Check sheet for the modelled part. Datum: model origin and axes. Units: mm. Face numbers are marked on the shaded views. Round coordinates to 2 decimals unless told otherwise and drop trailing zeros. Loops run counter-clockwise (first coordinate to the right, second up) from the corner with the lowest first, then second, coordinate; pieces in that order, holes last. Notation, with made-up numbers: (74.5, -8.5) -> (131.5, -8.5) arc R27 cw to (131.5, 20.5) -> close; hole circle Ø5 at (-20.5, 52). An arc over 180 degrees is marked (long way). One line per item, written item: value. Start each with the question number.
1. Material ranges on L1, parallel to X at y = 9, z = -64; L2, parallel to X at y = -8.5, z = -61.5; L3, parallel to Y at x = -8, z = -107.95, recorded low to high.
2. Cross-section at A-A on y = 54. Record the cut outline in (x, z), then the cut area to 3 significant figures.
3. Cross-section at B-B on y = 9. Record the cut outline in (x, z).
4. Release check for a two-part mould opening along X. For the marked faces 1, 2 and 3 record: +X half, -X half, draft (parallel to the pull), parting line (faces both ways), or undercut.
5. Go/stop test with flat-tipped pins: pin 1 (3 mm diameter, centred on y = 31, z = -119, fed in from +X); pin 2 (10 mm diameter, centred on x = 241.3, y = 0, fed in from -Z); pin 3 (8 mm diameter, centred on y = 50.5, z = -40, fed in from +X). Record where each tip stops, or that it passes through.
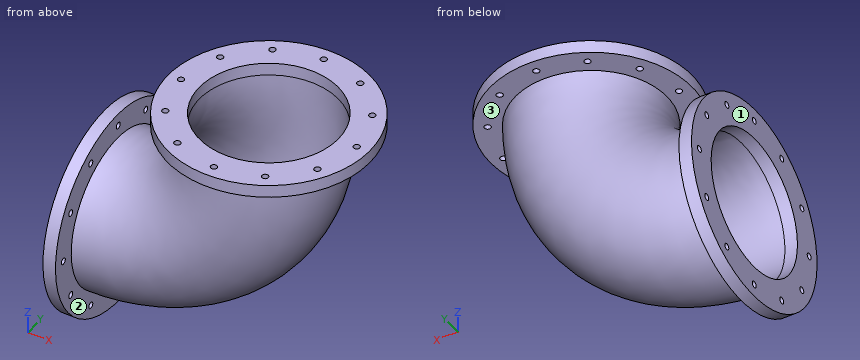
from build123d import *

# Parameters (mm, degrees)
SKETCH2_R           = 76.2
SKETCH2_R_2         = 69.85
SKETCH3_R           = 101.6
SKETCH3_R_2         = 69.85
SKETCH3_R_3         = 3.175
BOSS_EXTRUDE1_DEPTH = 12.7
SKETCH5_R           = 101.6
SKETCH5_R_2         = 69.85
SKETCH5_R_3         = 3.175
BOSS_EXTRUDE2_DEPTH = 12.7


with BuildPart() as part:
    # Sweep1: sweep along a path in Sketch1
    with BuildLine(Plane(origin=(0, 0, 0), x_dir=(1, 0, 0), z_dir=(0, 1, 0))) as sweep1_path:
        ThreePointArc((0, 152.4), (107.763073453, 107.763073453), (152.4, 0))
    # Sketch2 → Sweep1 (sweep)
    with BuildSketch(Plane(origin=(0, 0, 0), x_dir=(0, 0, -1), z_dir=(1, 0, 0))):
        with Locations((152.4, 0)):
            Circle(SKETCH2_R)
        with Locations((152.4, 0)):
            Circle(SKETCH2_R_2, mode=Mode.SUBTRACT)
    sweep(path=sweep1_path.line)

    # Sketch3 → Boss-Extrude1 (add)
    with BuildSketch(Plane.ZY):
        with Locations((-152.4, 0)):
            Circle(SKETCH3_R)
        with Locations((-152.4, 0)):
            Circle(SKETCH3_R_2, mode=Mode.SUBTRACT)
        with Locations((-241.3, 0)):
            Circle(SKETCH3_R_3, mode=Mode.SUBTRACT)
        with Locations((-229.389658396, -44.45)):
            Circle(SKETCH3_R_3, mode=Mode.SUBTRACT)
        with Locations((-196.85, -76.989658396)):
            Circle(SKETCH3_R_3, mode=Mode.SUBTRACT)
        with Locations((-152.4, -88.9)):
            Circle(SKETCH3_R_3, mode=Mode.SUBTRACT)
        with Locations((-107.95, -76.989658396)):
            Circle(SKETCH3_R_3, mode=Mode.SUBTRACT)
        with Locations((-75.410341604, -44.45)):
            Circle(SKETCH3_R_3, mode=Mode.SUBTRACT)
        with Locations((-63.5, 0)):
            Circle(SKETCH3_R_3, mode=Mode.SUBTRACT)
        with Locations((-75.410341604, 44.45)):
            Circle(SKETCH3_R_3, mode=Mode.SUBTRACT)
        with Locations((-107.95, 76.989658396)):
            Circle(SKETCH3_R_3, mode=Mode.SUBTRACT)
        with Locations((-152.4, 88.9)):
            Circle(SKETCH3_R_3, mode=Mode.SUBTRACT)
        with Locations((-196.85, 76.989658396)):
            Circle(SKETCH3_R_3, mode=Mode.SUBTRACT)
        with Locations((-229.389658396, 44.45)):
            Circle(SKETCH3_R_3, mode=Mode.SUBTRACT)
    extrude(amount=BOSS_EXTRUDE1_DEPTH)

    # Sketch5 → Boss-Extrude2 (add)
    with BuildSketch(Plane.XY):
        with Locations((152.4, 0)):
            Circle(SKETCH5_R)
        with Locations((152.4, 0)):
            Circle(SKETCH5_R_2, mode=Mode.SUBTRACT)
        with Locations((152.4, 88.9)):
            Circle(SKETCH5_R_3, mode=Mode.SUBTRACT)
        with Locations((196.85, 76.989658396)):
            Circle(SKETCH5_R_3, mode=Mode.SUBTRACT)
        with Locations((229.389658396, 44.45)):
            Circle(SKETCH5_R_3, mode=Mode.SUBTRACT)
        with Locations((241.3, 0)):
            Circle(SKETCH5_R_3, mode=Mode.SUBTRACT)
        with Locations((229.389658396, -44.45)):
            Circle(SKETCH5_R_3, mode=Mode.SUBTRACT)
        with Locations((196.85, -76.989658396)):
            Circle(SKETCH5_R_3, mode=Mode.SUBTRACT)
        with Locations((152.4, -88.9)):
            Circle(SKETCH5_R_3, mode=Mode.SUBTRACT)
        with Locations((107.95, -76.989658396)):
            Circle(SKETCH5_R_3, mode=Mode.SUBTRACT)
        with Locations((75.410341604, -44.45)):
            Circle(SKETCH5_R_3, mode=Mode.SUBTRACT)
        with Locations((63.5, 0)):
            Circle(SKETCH5_R_3, mode=Mode.SUBTRACT)
        with Locations((75.410341604, 44.45)):
            Circle(SKETCH5_R_3, mode=Mode.SUBTRACT)
        with Locations((107.95, 76.989658396)):
            Circle(SKETCH5_R_3, mode=Mode.SUBTRACT)
    extrude(amount=BOSS_EXTRUDE2_DEPTH)


solid = part.part
Taken from the geometry:
1. L1: x = -12.7 to 0, 42.33 to 53.06, 212.23 to 218.9
1. L2: x = -12.7 to 0, 45.79 to 55.84, 213.03 to 219.68
1. L3: y = -91.36 to -80.16, -73.81 to -53.88, 53.88 to 73.81, 80.16 to 91.36
2. outline: (-12.7, -238.46) -> (0, -238.46) -> (0, -206.16) arc R206.16 ccw to (206.16, 0) -> (238.46, 0) -> (238.46, 12.7) -> (196.71, 12.7) -> (196.71, 0) arc R196.71 cw to (0, -196.71) -> (-12.7, -196.71) -> close; (-12.7, -108.09) -> (0, -108.09) arc R108.09 ccw to (108.09, 0) -> (108.09, 12.7) -> (66.34, 12.7) -> (66.34, 0) -> (98.64, 0) arc R98.64 cw to (0, -98.64) -> (0, -66.34) -> (-12.7, -66.34) -> close
2. area: 6,650 mm2
3. outline: (-12.7, -253.6) -> (0, -253.6) -> (0, -228.07) arc R228.07 ccw to (228.07, 0) -> (253.6, 0) -> (253.6, 12.7) -> (221.67, 12.7) -> (221.67, 0) arc R221.67 cw to (0, -221.67) -> (-12.7, -221.67) -> close; (-12.7, -83.13) -> (0, -83.13) arc R83.13 ccw to (83.13, 0) -> (83.13, 12.7) -> (51.2, 12.7) -> (51.2, 0) -> (76.73, 0) arc R76.73 cw to (0, -76.73) -> (0, -51.2) -> (-12.7, -51.2) -> close
4. face 1: -X half
4. face 2: undercut
4. face 3: draft
5. pin 1: stops at x = 188.64
5. pin 2: stops at z = 0
5. pin 3: stops at x = 209.06
